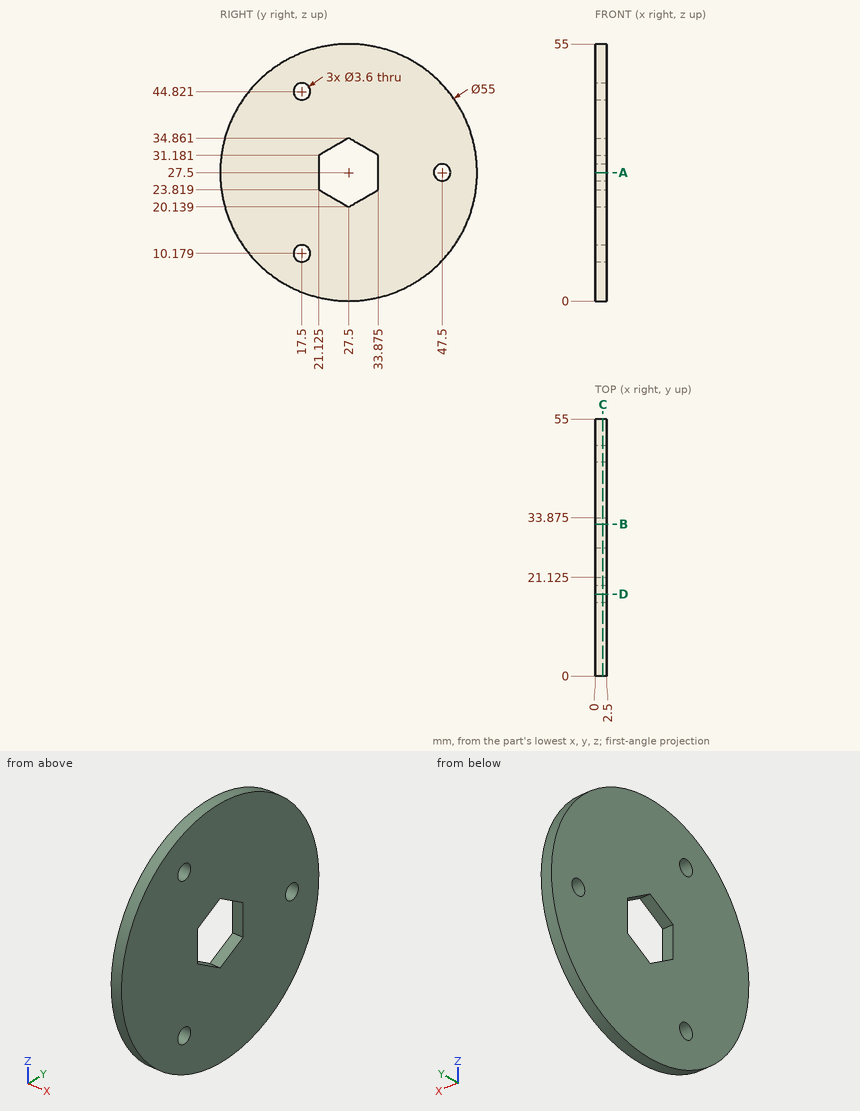
Can you work these out from the drawing? Everything is in mm from the part's minimum corner. Round coordinates to 2 decimals unless told otherwise and drop trailing zeros. Order: outer loops, then holes, each group sorted by start corner. A loop starts at its lowest first (then second) coordinate and runs counter-clockwise, first axis right, second up. Notation, with made-up numbers: (76, 58) -> (98, 58) arc R8 ccw to (98, 66) -> close; hole circle Ø8 at (68, 88). An arc over 180 degrees is marked (long way). Return JSON: item names as keys, results as strings. Group by question number.
1. If we section it at D-D, the plane y = 17.5: Write out the boundary of the cut face in (x, z), then the cut area to 3 significant figures.
2. Will these pins go through, and if not, where does the flat tip stop? pin 1 (10 mm diameter, centred on y = 33, z = 26, fed in from -X); pin 2 (1.2 mm diameter, centred on x = 1.5, z = 29, fed in from +Y) (1 decimal); pin 3 (1.2 mm diameter, centred on x = 1.5, z = 28, fed in from -Y); pin 4 (3 mm diameter, centred on y = 17.5, z = 10.18, fed in from -X).
3. If we section it at A-A, the plane z = 27.5: Write out the boundary of the cut face in (x, y) (1 decimal).
4. If we section it at B-B, the plane y = 32.5: Write out the boundary of the cut face in (x, z) (1 decimal), then the cut area to 3 significant figures.
5. I need wall thicknesses on line 1 (Y direction, x = 1.75, z = 27.5) (1 decimal); line 2 (Z direction, x = 2.2, y = 18); line 3 (Y direction, x = 0.4, z = 27) (1 decimal). Which ranges of each line are inside material? Lowest first, please. Write a range as [from, to].
6. If we section it at C-C, the plane x = 1.65: Write out the boundary of the cut face in (y, z) (1 decimal).
Output values:
{
 "1": {"outline": "(0, 1.88) -> (2.5, 1.88) -> (2.5, 8.38) -> (0, 8.38) -> close; (0, 11.98) -> (2.5, 11.98) -> (2.5, 43.02) -> (0, 43.02) -> close; (0, 46.62) -> (2.5, 46.62) -> (2.5, 53.12) -> (0, 53.12) -> close", "area": "110 mm²"},
 "2": {"pin 1": "x = 0", "pin 2": "y = 55", "pin 3": "y = 0", "pin 4": "through"},
 "3": {"outline": "(0, 0) -> (2.5, 0) -> (2.5, 21.1) -> (0, 21.1) -> close; (0, 33.9) -> (2.5, 33.9) -> (2.5, 45.7) -> (0, 45.7) -> close; (0, 49.3) -> (2.5, 49.3) -> (2.5, 55) -> (0, 55) -> close"},
 "4": {"outline": "(0, 0.5) -> (2.5, 0.5) -> (2.5, 23) -> (0, 23) -> close; (0, 32) -> (2.5, 32) -> (2.5, 54.5) -> (0, 54.5) -> close", "area": "113 mm²"},
 "5": {"line 1": "[0, 21.1], [33.9, 45.7], [49.3, 55]", "line 2": "[1.69, 8.45], [11.91, 43.09], [46.55, 53.31]", "line 3": "[0, 21.1], [33.9, 45.8], [49.2, 55]"},
 "6": {"outline": "circle Ø55 at (27.5, 27.5); hole circle Ø3.6 at (17.5, 10.2); hole circle Ø3.6 at (17.5, 44.8); hole (21.1, 23.8) -> (27.5, 20.1) -> (33.9, 23.8) -> (33.9, 31.2) -> (27.5, 34.9) -> (21.1, 31.2) -> close; hole circle Ø3.6 at (47.5, 27.5)"}
}
